Can you work these out from the model? Positions are in its coordinate system, mm. Face numbers are marked on the shaded views. Give positions to 0.01 mm unless a question says otherwise; leave off trailing zeros. Write each loop counter-clockwise with the first axis right and the second up, starting at its lowest first coordinate (ties: lowest second). Pieces come first, ordered by that corner, then holes.
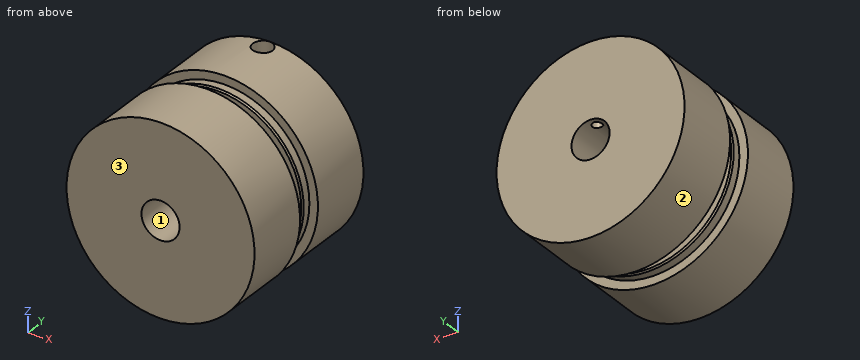
```python
from build123d import *

# Parameters (mm, degrees)
F2_SIZE        = 0.762
F3_R           = 0.254
F6_D           = 5.1054
F6_DEPTH       = 49.3522
F6_START       = 0.2754562
F6_CBORE_D     = 10.414
F6_CBORE_DEPTH = 33.4772
F6_TIP         = 1.5338169022


with BuildPart() as f1:
    # F0 (on Right) → F1 (revolve)
    with BuildSketch(Plane.YZ):
        Polygon((-41.4782, 10.0076), (0, 10.0076), (41.4782, 10.0076), (41.4782, 49.3522), (6.7945, 49.3522), (6.7945, 44.8818), (1.7145, 44.8818), (1.7145, 32.1818), (-1.7145, 32.1818), (-1.7145, 44.8818), (-6.7945, 44.8818), (-6.7945, 49.3522), (-41.4782, 49.3522), align=None)
    revolve(axis=Axis((0, -0.9843776588, 0), (0, 1, 0)))

    # F2
    f2_edges = [f1.edges().sort_by_distance(p)[0] for p in [
        (0, 1.7145, -44.8818),
        (0, -1.7145, -44.8818),
    ]]
    chamfer(f2_edges, length=F2_SIZE)

    # F3
    f3_edges = [f1.edges().sort_by_distance(p)[0] for p in [
        (0, -1.7145, -32.1818),
        (0, 1.7145, -32.1818),
    ]]
    fillet(f3_edges, radius=F3_R)

    # F6
    # its depths count from where the whole tool has entered the part; down to there all is cleared
    with Locations(Plane.XY.offset(49.3522).offset(-F6_START)):
        with Locations((0, 36.2458)):
            CounterBoreHole(F6_D / 2, F6_CBORE_D / 2, F6_CBORE_DEPTH, depth=F6_DEPTH)
            with Locations((0, 0, -(F6_DEPTH + F6_TIP / 2))):  # 118° drill point
                Cone(0, F6_D / 2, F6_TIP, mode=Mode.SUBTRACT)


solid = f1.part
```
1) Suppose I cut it at B-B on y = -32. Write out the boundary of the cut face in (x, z).
Values follow:
outline: circle Ø98.7 at (0, 0); hole circle Ø20.02 at (0, 0)
2) If we mould it in two halves opening along X, with no side actions, what happens to the marked faces 1, 2 and 3? For each: +X half, -X half, draft (parallel to the pull), parting line (faces both ways), or undercut.
Values follow:
face 1: undercut
face 2: parting line
face 3: draft
3) Suppose I cut it at C-C on x = 0. State how many separate pieces and enclosed holes the cut face has, plus the area to 3 significant figures.
Values follow:
separate pieces: 3
enclosed holes: 0
area: 5,940 mm2
4) For pin 1 Ø6 at (y, z) = (-11, -21.5) entering from +X; pin 2 Ø1 at (y, z) = (-31, -14) entering from +X; pin 3 Ø5 at (y, z) = (-3.5, 25.5) entering from +X, each with a flat end and sliding along its axis, tell me the tip position at first contact or that it passes through.
Values follow:
pin 1: stops at x = 45.75
pin 2: stops at x = 47.47
pin 3: stops at x = 38.54
5) Please list where these lines run through material, in increasing order: L1, parallel to Y at x = 0, z = 13; L2, parallel to X at y = -23, z = 0; L3, parallel to Y at x = -32, z = 17.
Values follow:
L1: y = -41.48 to 33.69, 38.8 to 41.48
L2: x = -49.35 to -10.01, 10.01 to 49.35
L3: y = -41.48 to -1.71, 1.71 to 41.48
